```python
from build123d import *

# Parameters (mm, degrees)
F0_R     = 11.049
F1_DEPTH = 6.35
F2_R     = 3.17499


# Not quite as in the source:
# - a fillet or chamfer is up to 0.001 mm smaller than in the source, because OpenCascade refuses the exact size


with BuildPart() as f1:
    # F0 (on Top) → F1 (new body)
    with BuildSketch(Plane.XY):
        with BuildLine():
            ThreePointArc((10.266368543, 9.474311423), (5.6037830713, 12.7968166076), (0, 13.97))
            ThreePointArc((0, 13.97), (-5.3724040771, 12.8956649473), (-9.9185000629, 9.8378989882))
            ThreePointArc((-9.9185000629, 9.8378989882), (-10.4709665549, 9.247689409), (-10.9883672437, 8.6265106107))
            Line((-10.9883672437, 8.6265106107), (-14.8673558727, 10.7216511471))
            Line((-14.8673558727, 10.7216511471), (-18.2652639065, 21.743875915))
            Line((-18.2652639065, 21.743875915), (-20.7996486885, 21.3214784899))
            Line((-20.7996486885, 21.3214784899), (-18.0642706589, 12.4483862321))
            Line((-18.0642706589, 12.4483862321), (-27.1912532422, 17.3781019425))
            Line((-27.1912532422, 17.3781019425), (-28.7577700617, 14.4778187277))
            Line((-28.7577700617, 14.4778187277), (-19.9750544664, 9.7340503842))
            Line((-19.9750544664, 9.7340503842), (-27.5974388749, 8.4636530986))
            Line((-27.5974388749, 8.4636530986), (-27.1215043395, 5.6080456262))
            Line((-27.1215043395, 5.6080456262), (-15.8225889535, 7.4911980188))
            Line((-15.8225889535, 7.4911980188), (-12.7056009028, 5.8076333991))
            ThreePointArc((-12.7056009028, 5.8076333991), (-13.0481194381, 4.9907393369), (-13.3381786472, 4.1537802513))
            ThreePointArc((-13.3381786472, 4.1537802513), (-12.2222121685, -6.7659758874), (-3.5606204122, -13.508622516))
            ThreePointArc((-3.5606204122, -13.508622516), (-2.773250677, -13.6919677433), (-1.9765937131, -13.8294604845))
            Line((-1.9765937131, -13.8294604845), (-1.8515443275, -18.2363334465))
            Line((-1.8515443275, -18.2363334465), (-9.6981169659, -26.6901205073))
            Line((-9.6981169659, -26.6901205073), (-8.0651176742, -28.6737633989))
            Line((-8.0651176742, -28.6737633989), (-1.7484833836, -21.8683104075))
            Line((-1.7484833836, -21.8683104075), (-1.4542511306, -32.2373670397))
            Line((-1.4542511306, -32.2373670397), (1.8407262213, -32.1438687935))
            Line((1.8407262213, -32.1438687935), (1.5575923187, -22.165929802))
            Line((1.5575923187, -22.165929802), (6.4689808452, -28.1319096943))
            Line((6.4689808452, -28.1319096943), (8.7040421919, -26.29193456))
            Line((8.7040421919, -26.29193456), (1.4237266877, -17.4483629968))
            Line((1.4237266877, -17.4483629968), (1.323242392, -13.9071898517))
            ThreePointArc((1.323242392, -13.9071898517), (2.2019526696, -13.7953725735), (3.0718101042, -13.6280916743))
            ThreePointArc((3.0718101042, -13.6280916743), (11.9706130841, -7.2017582846), (13.4791204751, 3.6707235278))
            ThreePointArc((13.4791204751, 3.6707235278), (13.244217232, 4.4442783342), (12.9649609568, 5.2029498738))
            Line((12.9649609568, 5.2029498738), (16.7189002003, 7.5146822993))
            Line((16.7189002003, 7.5146822993), (27.9633808724, 4.9462445923))
            Line((27.9633808724, 4.9462445923), (28.8647663627, 7.3522849091))
            Line((28.8647663627, 7.3522849091), (19.8127540426, 9.4199241754))
            Line((19.8127540426, 9.4199241754), (28.6455043728, 14.8592650972))
            Line((28.6455043728, 14.8592650972), (26.9170438404, 17.6660500658))
            Line((26.9170438404, 17.6660500658), (18.9289850868, 12.7468829615))
            Line((18.9289850868, 12.7468829615), (18.4174621476, 12.4318794178))
            Line((18.4174621476, 12.4318794178), (21.1284580297, 19.6682565957))
            Line((21.1284580297, 19.6682565957), (18.4174621476, 20.6838889338))
            Line((18.4174621476, 20.6838889338), (14.3988622659, 9.957164978))
            Line((14.3988622659, 9.957164978), (11.3823585109, 8.0995564527))
            ThreePointArc((11.3823585109, 8.0995564527), (10.8461667685, 8.8046332365), (10.266368543, 9.474311423))
        make_face()
        with BuildLine():
            ThreePointArc((0, 11.049), (7.8128228253, 7.8128228253), (11.049, 0))
            ThreePointArc((11.049, 0), (-7.8128228253, -7.8128228253), (0, 11.049))
        make_face(mode=Mode.SUBTRACT)
        with BuildLine():
            ThreePointArc((-9.9185000629, 9.8378989882), (-5.3724040771, 12.8956649473), (0, 13.97))
            ThreePointArc((0, 13.97), (5.6037830713, 12.7968166076), (10.266368543, 9.474311423))
            Line((10.266368543, 9.474311423), (12.8332442979, 14.8954782635))
            Line((12.8332442979, 14.8954782635), (15.1805052923, 35.3235639632))
            Line((15.1805052923, 35.3235639632), (0, 50.6446287036))
            Line((0, 50.6446287036), (-15.4629256576, 35.3235639632))
            Line((-15.4629256576, 35.3235639632), (-12.0582450181, 14.8954782635))
            Line((-12.0582450181, 14.8954782635), (-9.9185000629, 9.8378989882))
        make_face()
        with BuildLine():
            ThreePointArc((11.049, 27.94), (7.8128228253, 20.1271771747), (0, 16.891))
            ThreePointArc((0, 16.891), (-7.8128228253, 35.7528228253), (11.049, 27.94))
        make_face(mode=Mode.SUBTRACT)
        with BuildLine():
            ThreePointArc((-3.5606204122, -13.508622516), (-12.2222121685, -6.7659758874), (-13.3381786472, 4.1537802513))
            Line((-13.3381786472, 4.1537802513), (-19.3164847266, 3.6661764432))
            Line((-19.3164847266, 3.6661764432), (-38.1813563905, -4.5150787562))
            Line((-38.1813563905, -4.5150787562), (-43.8595350225, -25.3223143518))
            Line((-43.8595350225, -25.3223143518), (-22.8596409155, -31.0530684179))
            Line((-22.8596409155, -31.0530684179), (-6.8707400686, -17.8904856425))
            Line((-6.8707400686, -17.8904856425), (-3.5606204122, -13.508622516))
        make_face()
        with Locations((-24.1967497817, -13.97)):
            Circle(F0_R, mode=Mode.SUBTRACT)
        with BuildLine():
            Line((18.9289850868, 2.995007379), (13.4791204751, 3.6707235278))
            ThreePointArc((13.4791204751, 3.6707235278), (11.9706130841, -7.2017582846), (3.0718101042, -13.6280916743))
            Line((3.0718101042, -13.6280916743), (6.4832404288, -18.5616547067))
            Line((6.4832404288, -18.5616547067), (23.0008510982, -30.808485207))
            Line((23.0008510982, -30.808485207), (43.8595350225, -25.3223143518))
            Line((43.8595350225, -25.3223143518), (38.3225665731, -4.2704955452))
            Line((38.3225665731, -4.2704955452), (18.9289850868, 2.995007379))
        make_face()
        with Locations((24.1967497817, -13.97)):
            Circle(F0_R, mode=Mode.SUBTRACT)
    extrude(amount=F1_DEPTH)

    # F2 (radius 3.175 in the source; OpenCascade refuses exactly that, so slightly less here)
    f2_edges = [f1.edges().sort_by_distance(p)[0] for p in [
        (-7.731463, 42.984096, 6.35),
        (7.590253, 42.984096, 6.35),
        (41.091051, -14.796405, 6.35),
        (33.430193, -28.0654, 6.35),
        (-41.020446, -14.918697, 6.35),
        (-33.359588, -28.187691, 6.35),
        (-33.359588, -28.187691, 0),
        (-41.020446, -14.918697, 0),
        (-7.731463, 42.984096, 0),
        (41.091051, -14.796405, 0),
        (33.430193, -28.0654, 0),
    ]]
    fillet(f2_edges, radius=F2_R)


solid = f1.part
```
Source: CAD feature listing. Evaluate the final solid. Frame: model axes, mm. A direction names the side the tool comes from. Round coordinates to 2 decimals unless told otherwise and drop trailing zeros. Loops run counter-clockwise (first coordinate to the right, second up) from the corner with the lowest first, then second, coordinate; pieces in that order, holes last. Notation, with made-up numbers: (-34, -37.5) - (23, -37.5) arc R23 ccw to (23, -2.5) - close; hole circle Ø3 at (69.25, -38.5). An arc over 180 degrees is marked (long way). Use CSV: the item, a comma, the result in double quotes.
Q1. Mould query, pull axis X, two halves, no side actions, for faces 1 (the cylindrical face through (32.133, -27.47, 5.395)), 2 (the flat face through (-28.62, -0.37, 3.13)), 3 (the flat face through (-14.977, -24.564, 3.131)), 4 (the flat face through (3.98, -25.11, 3.13)). Classes: pulls with the +X half, pulls with the -X half, needs draft (parallel to the pull), parting line crosses it, or undercut.
Reported:
face 1,"pulls with the +X half"
face 2,"pulls with the -X half"
face 3,"undercut"
face 4,"undercut"
Q2. Pin query (flat end, axial travel): pin 1 Ø2 at (x, z) = (-16.5, 2.5) entering from -Y; pin 2 Ø1 at (x, z) = (-19, 5.5) entering from +Y. Return the tip coordinate at first contact, or that it passes through.
Reported:
pin 1,"y = -26.64"
pin 2,"y = 21.7"
Q3. Reachability of faces 5 (the flat face through (24.402, 8.372, 3.131)), 6 (the flat face through (22.26, 6.25, 3.13)), 7 (the flat face through (-16.285, 3.913, 3.131)) from +Z, -Z, +X, -X, +Y, -Y: full face, straight path, thin tool, end or side. Return the list, or none.
Reported:
face 5,"+Z, -Z, +X"
face 6,"+Z, -Z"
face 7,"+Z, -Z, -X"
Q4. Ray query, line 1 along X through (y, z) = (-7, 0.5); line 2 along Y through (x, z) = (-26.5, 2); line 3 along Y through (x, z) = (10, 2). Return the intervals inside material, ascending.
Reported:
line 1,"-37.34 to -32.77, -15.62 to -8.55, 8.55 to 15.62, 32.77 to 37.53"
line 2,"-29.83 to -24.78, -3.16 to 0.55, 5.71 to 8.65, 13.26 to 17"
line 3,"-21.17 to -4.7, 4.7 to 23.24, 32.64 to 40.55"
Q5. Section query A-A, the plane y = 26. Output: boundary loops of the cut face in (x, z).
Reported:
outline,"(-13.91, 0) - (-10.88, 0) - (-10.88, 6.35) - (-13.91, 6.35) - close; (10.88, 0) - (14.11, 0) - (14.11, 6.35) - (10.88, 6.35) - close"
